from build123d import *

# Parameters (mm, degrees)
F1_DEPTH  = 40
F2_W      = 30
F2_H      = 45
F3_DEPTH  = 4
F5_DEPTH  = 45.001
F7_DEPTH  = 42.001
F9_DEPTH  = 30.001
F11_DEPTH = 5
F12_R     = 0.5


with BuildPart() as f1:
    # F0 (on Top) → F1 (new body)
    with BuildSketch(Plane.XY):
        Polygon((0, 0), (30, 0), (30, 8), (25, 8), (25, 5), (27, 5), (27, 3), (3, 3), (3, 42), (5, 42), (5, 40), (8, 40), (8, 45), (0, 45), align=None)
    extrude(amount=F1_DEPTH)

    # F2 (on Top) → F3 (join)
    with BuildSketch(Plane.XY):
        with Locations((15, 22.5)):
            Rectangle(F2_W, F2_H)
    extrude(amount=-F3_DEPTH)

    # F4 (on Front) → F5 (cut, through all)
    with BuildSketch(Plane.XZ):
        Polygon((18, 0), (30, 0), (30, 11.40249), (18, 3), align=None)
    extrude(amount=-F5_DEPTH, mode=Mode.SUBTRACT)

    # F6 (on face) → F7 (cut, through all)
    with BuildSketch(Plane(origin=(0, 3, 0), x_dir=(-1, 0, 0), z_dir=(0, 1, 0))):
        Polygon((-18, 3), (-18, 19.804981), (-30, 11.40249), (-30, 3), align=None)
    extrude(amount=F7_DEPTH, mode=Mode.SUBTRACT)

    # F8 (on Right) → F9 (cut, through all)
    with BuildSketch(Plane.YZ):
        Polygon((33, 0), (45, 0), (45, 11.40249), (33, 3), align=None)
    extrude(amount=F9_DEPTH, mode=Mode.SUBTRACT)

    # F10 (on face) → F11 (cut, through all)
    with BuildSketch(Plane.YZ.offset(8)):
        Polygon((40, 7.901453), (45, 11.40249), (40, 14.289242), align=None)
    extrude(amount=-F11_DEPTH, mode=Mode.SUBTRACT)

    # F12
    f12_edges = [f1.edges().sort_by_distance(p)[0] for p in [
        (0, 45, 25.701245),
        (0, 45, -2),
        (0, 0, 18),
        (30, 0, 25.701245),
        (30, 0, -2),
        (30, 8, 25.701245),
        (8, 40, 27.144621),
        (8, 45, 25.701245),
        (30, 22.5, 0),
        (30, 22.5, -4),
        (15, 45, 0),
        (15, 45, -4),
        (30, 45, -2),
        (25, 8, 27.451764),
        (15, 0, -4),
        (0, 22.5, -4),
        (3, 3, 20),
    ]]
    fillet(f12_edges, radius=F12_R)


solid = f1.part
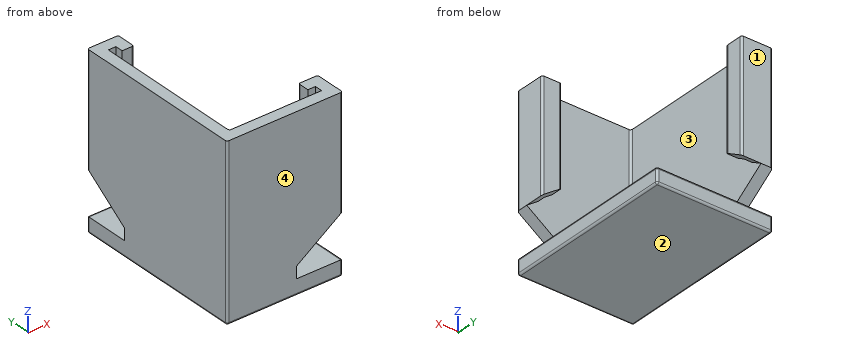
The listing builds one solid part. Answer for the finished solid, in the listing's coordinates (mm). Face numbers are marked on the shaded views. Give positions to 0.01 mm unless a question says otherwise; leave off trailing zeros. Loops run counter-clockwise (first coordinate to the right, second up) from the corner with the lowest first, then second, coordinate; pieces in that order, holes last. Notation, with made-up numbers: (-14.5, 66) - (-4.5, 66) arc R16 cw to (-4.5, 83) - close; hole circle Ø3 at (15.25, 36). An arc over 180 degrees is marked (long way). Answer as a JSON object with one key per item and string values.
1. A cutting plane is placed at C-C (y = 34). Write down the section's boundary in (x, z), then the cut area to 3 significant figures.
Determined:
{"outline": "(0, -3.5) arc R0.5 ccw to (0.5, -4) - (29.5, -4) arc R0.5 ccw to (30, -3.5) - (30, -0.5) arc R0.5 ccw to (29.5, 0) - (0, 0) - close; (0, 3.7) - (3, 3.7) - (3, 40) - (0, 40) - close", "area": "229 mm²"}
2. A cutting plane is placed at A-A (z = 28.5). Write down the section's boundary in (x, y).
Determined:
{"outline": "(0, 0.5) arc R0.5 ccw to (0.5, 0) - (29.5, 0) arc R0.5 ccw to (30, 0.5) - (30, 7.5) arc R0.5 ccw to (29.5, 8) - (25.5, 8) arc R0.5 ccw to (25, 7.5) - (25, 5) - (27, 5) - (27, 3) - (3.5, 3) arc R0.5 cw to (3, 3.5) - (3, 42) - (5, 42) - (5, 40) - (7.5, 40) arc R0.5 ccw to (8, 40.5) - (8, 44.5) arc R0.5 ccw to (7.5, 45) - (0.5, 45) arc R0.5 ccw to (0, 44.5) - close"}
3. A cutting plane is placed at B-B (x = 11.75). Write down the section's boundary in (y, z), then the cut area to 3 significant figures.
Determined:
{"outline": "(0, -3.5) arc R0.5 ccw to (0.5, -4) - (44.5, -4) arc R0.5 ccw to (45, -3.5) - (45, -0.5) arc R0.5 ccw to (44.5, 0) - (3, 0) - (3, 40) - (0, 40) - close", "area": "300 mm²"}
4. For a pull along Y with two mould halves and no side action, classify the marked faces 1, 2, 3 and 4 as pulls with the +Y half, pulls with the -Y half, needs draft (parallel to the pull), parting line crosses it, or undercut.
Determined:
{"face 1": "pulls with the +Y half", "face 2": "needs draft", "face 3": "undercut", "face 4": "pulls with the -Y half"}
5. Find the intervals of material crossed by L1, parallel to Y at x = 7.5, z = 31; L2, parallel to Y at x = 25.5, z = 35; L3, parallel to X at y = 4.5, z = 25, in increasing order. Write a range as [from, to].
Determined:
{"L1": "[0, 3], [40, 45]", "L2": "[0, 3], [5, 8]", "L3": "[0, 3], [27, 30]"}
6. A cutting plane is placed at D-D (y = 28). Write down the section's boundary in (x, z).
Determined:
{"outline": "(0, -3.5) arc R0.5 ccw to (0.5, -4) - (29.5, -4) arc R0.5 ccw to (30, -3.5) - (30, -0.5) arc R0.5 ccw to (29.5, 0) - (3, 0) - (3, 40) - (0, 40) - close"}
7. Flat-ended cylindrical pins translate along their axes: pin 1 Ø4.5 at (y, z) = (43, 32) entering from +X; pin 2 Ø6 at (x, y) = (17, 8.5) entering from +Z; pin 3 Ø1.2 at (x, z) = (26.5, 26.5) entering from +Y. Find the tip coordinate at first contact, or state that the pin passes through.
Determined:
{"pin 1": "x = 8", "pin 2": "z = 0", "pin 3": "y = 8"}
